```python
from build123d import *

# Parameters (mm, degrees)
F0_W     = 67.9279565811
F0_H     = 88.0647003651
F1_DEPTH = 25.4
F1_TAPER = 3


# Not quite as in the source:
# - a feature of the source that left no trace in its solid (it failed there, or was rolled back) is left out


with BuildPart() as f1:
    # F0 (on Top) → F1 (new body)
    with BuildSketch(Plane.XY):
        Rectangle(F0_W, F0_H)
    extrude(amount=F1_DEPTH, taper=F1_TAPER)

    # F2 (on Front) → F3 (revolve)
    with BuildSketch(Plane.XZ):
        Polygon((13.9438202605, 97.8820249438), (13.9438202605, 0), (62.8700107336, 0), (62.8700107336, 8.7491702288), (22.6633418351, 8.7491702288), (22.6633418351, 28.8525056094), (48.57968539, 28.8525056094), (48.57968539, 51.3779297471), (30.8984406292, 51.3779297471), (30.8984406292, 63.9727860689), (48.3374781907, 62.0351172984), (48.3374781907, 68.8169673085), (35.5004072189, 68.8169673085), (46.6420166194, 86.0137939453), (23.8743834198, 86.0137939453), (23.8743834198, 97.8820249438), align=None)
    revolve(axis=Axis((-40, 0, 38.2511918375), (0, 0, 1)))


solid = f1.part
```
Input: part model. Units: mm. Frame: model coordinates. A direction names the side the tool comes from. Give positions to 0.01 mm unless a question says otherwise; leave off trailing zeros. Write each loop counter-clockwise with the first axis right and the second up, starting at its lowest first coordinate (ties: lowest second). Pieces come first, ordered by that corner, then holes. Notation, with made-up numbers: (10.5, 63) - (16.5, 63) arc R19 cw to (16.5, 100) - close; hole circle Ø11 at (1, 66). An arc over 180 degrees is marked (long way). Write item = value, one per line. Start each with the question number.
1. Section query A-A, the plane z = 45. Output: boundary loops of the cut face in (x, y), then the cut area to 3 significant figures.
2. Section query C-C, the plane z = 56.5. Output: boundary loops of the cut face in (x, y), then the cut area to 3 significant figures.
3. Access query for faces 1 (the cylindrical face through (44.49, 26.61, 40.27)), 2 (the flat face through (19.07, 43.144, 16.958)), 3 (the conical face through (-56.518, -74.385, 69.893)), 4 (the flat face through (25, 1, 25.4)), 5 (the flat face through (19.469, -43.144, 16.958)). Directions: +Z, -Z, +X, -X, +Y, -Y. A direction counts if a zero-diameter tool reaches every point of the face in a straight line with its end or side. Return the directions, or none.
4. Mould query, pull axis Y, two halves, no side actions, for faces 6 (the cylindrical face through (-59.15, -86.237, 65.474)), 7 (the flat face through (-80, 59, 51.378)), 8 (the flat face through (-33.308, -0.616, 12.522)). Classes: released by +Y, released by -Y, zero draft, split by the parting line, or undercut.
5. Ray query, L1, parallel to Z at x = -51.5, y = -70; L2, parallel to Y at x = -40, z = 66.5; L3, parallel to Z at x = -13.5, y = -69.5. Return the intervals inside material, ascending.
6. Section query D-D, the plane z = 12. Output: boundary loops of the cut face in (x, y).
7. First-contact query: pin 1 Ø10 at (x, z) = (-21.5, 79) entering from -Y; pin 2 Ø5 at (x, z) = (19, 57) entering from +Y; pin 3 Ø5 at (x, z) = (-69, 28) entering from +Y. Flat tips, straight axial feed; report the tip coordinate or a pass-through.
Check sheet entries:
q1.outline = circle Ø177.16 at (-40, 0); hole circle Ø107.89 at (-40, 0)
q1.area = 15,500 mm2
q2.outline = circle Ø141.8 at (-40, 0); hole circle Ø107.89 at (-40, 0)
q2.area = 6,650 mm2
q3.face_1 = +Z
q3.face_2 = +X, +Y
q3.face_3 = none
q3.face_4 = +X
q3.face_5 = +X, -Y
q4.face_6 = split by the parting line
q4.face_7 = zero draft
q4.face_8 = undercut
q5.L1 = 0 to 8.75, 28.85 to 51.38, 63.97 to 86.01
q5.L2 = -88.34 to -53.94, 53.94 to 88.34
q5.L3 = 0 to 8.75, 28.85 to 51.38, 63.59 to 86.01
q6.outline = (5.2, -43.4) - (33.34, -43.4) - (33.34, 43.4) - (5.2, 43.4) arc R62.66 ccw (long way) to start; hole (-33.34, -43.4) - (-33.34, 43.4) - (-7.97, 43.4) arc R53.94 ccw (long way) to (-7.97, -43.4) - close
q7.pin_1 = -83.47
q7.pin_2 = 42.83
q7.pin_3 = 84.48
